Part model, mm, in its own coordinate system. A direction names the side the tool comes from. Give positions to 0.01 mm unless a question says otherwise; leave off trailing zeros. Order: outer loops, then holes, each group sorted by start corner. A loop starts at its lowest first (then second) coordinate and runs counter-clockwise, first axis right, second up. Notation, with made-up numbers: (50.5, 67) -> (76.5, 67) arc R20 cw to (76.5, 102) -> close; hole circle Ø7 at (15, 45). An arc over 180 degrees is marked (long way). Write item = value, one per line. Start each with the question number.
Item 1: Flat gauge pin, fed straight in: P1, Ø1, axis at x = -6, z = 1, coming from the -Y side. Where does the tip first touch, or does it go through?
Item 2: Band-saw the part on B-B on y = 1.5. Write the cut outline in (x, z).
Item 3: Pull direction Y, two halves, no side cores. Call faces 1 (the face through (-4.776, 1.007, 0.986)), 2 (the face through (1, -5, 1)), 3 (the face through (17.5, 0, 1)): +Y half, -Y half, draft (parallel to the pull), parting line (faces both ways), or undercut.
Item 4: Drill centre lines: line 1 along Y through (x, z) = (-7, 0.45); line 2 along Y through (x, z) = (-4, 1.95); line 3 along X through (y, z) = (-9.25, 1.45). Where is each one in solid material? Low to high.
Item 5: Band-saw the part on A-A on y = -2.5. Write the cut outline in (x, z), plus the area to 3 significant figures.
Item 6: Band-saw the part on C-C on x = 4. Write the cut outline in (y, z).
Item 7: Band-saw the part on D-D on y = -0.5. Write the cut outline in (x, z), plus the area to 3 significant figures.
Item 8: Tool access for faces 4 (the face through (3.224, 1.007, 0.986)), 5 (the face through (-17.5, -9, 1)): list every direction of +Z, -Z, +X, -X, +Y, -Y with a clear straight run to the whole face (end or side of a thin tool).
```python
from build123d import *

# Parameters (mm, degrees)
EXTRUDE_1_DEPTH = 2
HOLE_WIZARD_1_D = 3
HOLE_WIZARD_2_D = 3


with BuildPart() as part:
    # 草图1 → 凸台-拉伸1 (new body)
    with BuildSketch(Plane.XY):
        with BuildLine():
            Line((17.5, 5), (-17.5, 5))
            Line((-17.5, 5), (-21.5, 5))
            ThreePointArc((-21.5, 5), (-25.742640687, 3.242640687), (-27.5, -1))
            Line((-27.5, -1), (-27.5, -10))
            Line((-27.5, -10), (-17.5, -10))
            Line((-17.5, -10), (-17.5, -8))
            ThreePointArc((-17.5, -8), (-16.621320344, -5.878679656), (-14.5, -5))
            Line((-14.5, -5), (17.5, -5))
            Line((17.5, -5), (17.5, 5))
        make_face()
    extrude(amount=EXTRUDE_1_DEPTH)

    # 孔1 (through all)
    with Locations(Plane.XY.offset(2)):
        with Locations((-22.498361417, -1.410422078)):
            Hole(HOLE_WIZARD_1_D / 2)

    # 孔2 (through all)
    with Locations(Plane.XY.offset(2)):
        with Locations((4.655, 0.556399926), (-3.345, 0.556399926)):
            Hole(HOLE_WIZARD_2_D / 2)


solid = part.part
```
Values found:
q1.P1 = -5
q2.outline = (-26.95, 0) -> (-4.51, 0) -> (-4.51, 2) -> (-26.95, 2) -> close; (-2.18, 0) -> (3.49, 0) -> (3.49, 2) -> (-2.18, 2) -> close; (5.82, 0) -> (17.5, 0) -> (17.5, 2) -> (5.82, 2) -> close
q3.face_1 = undercut
q3.face_2 = -Y half
q3.face_3 = draft
q4.line_1 = -5 to 5
q4.line_2 = -5 to -0.79, 1.91 to 5
q4.line_3 = -27.5 to -17.5
q5.outline = (-27.5, 0) -> (-23.53, 0) -> (-23.53, 2) -> (-27.5, 2) -> close; (-21.47, 0) -> (17.5, 0) -> (17.5, 2) -> (-21.47, 2) -> close
q5.area = 85.9 mm^2
q6.outline = (-5, 0) -> (-0.79, 0) -> (-0.79, 2) -> (-5, 2) -> close; (1.91, 0) -> (5, 0) -> (5, 2) -> (1.91, 2) -> close
q7.outline = (-27.48, 0) -> (-23.69, 0) -> (-23.69, 2) -> (-27.48, 2) -> close; (-21.31, 0) -> (-4.41, 0) -> (-4.41, 2) -> (-21.31, 2) -> close; (-2.28, 0) -> (3.59, 0) -> (3.59, 2) -> (-2.28, 2) -> close; (5.72, 0) -> (17.5, 0) -> (17.5, 2) -> (5.72, 2) -> close
q7.area = 76.7 mm^2
q8.face_4 = +Z, -Z
q8.face_5 = +Z, -Z, +X, -Y
